Could you check a few things on this model? Use its own coordinates, in mm. Face numbers are marked on the shaded views. A direction names the side the tool comes from. Give positions to 0.01 mm unless a question says otherwise; leave off trailing zeros. Write each loop counter-clockwise with the first axis right and the second up, starting at its lowest first coordinate (ties: lowest second). Pieces come first, ordered by that corner, then holes. Notation, with made-up numbers: (48.5, 9.25) - (71.5, 9.25) arc R23 cw to (71.5, 42.25) - close; hole circle Ø7 at (70, 23). An arc over 180 degrees is marked (long way). Answer as CSV lines item,"result". Start each with the question number.
Q1. Imagine slicing it at B-B on x = 23. List the corners of the cut face in (y, z) for me.
Q2. Imagine slicing it at A-A on z = 7.9. List the corners of the cut face in (x, y) for me.
Q3. We'd pull the mould along X, two halves only. Please class the marked faces 4, 5, 6 and 7: pulls with the +X half, pulls with the -X half, needs draft (parallel to the pull), parting line crosses it, or undercut.
Q4. On a 3-axis mill with a long thin cutter (end or side, diameter ignored), from which of +Z, -Z, +X, -X, +Y, -Y can I reach the whole of each face in a straight line? I mean the marked faces 1, 2 and 3. Say none if no direction works.
Q5. Imagine slicing it at D-D on z = -4. List the corners of the cut face in (x, y) for me, and give its area (3 significant figures).
Q6. If I drill on line 1 along Z through (x, y) = (20, -7); line 2 along X through (y, z) = (-11, 9); line 3 along Y through (x, z) = (12.5, 0.5), over which ranges is the centre line in solid material (lowest first)?
Q7. Will these pins go through, and if not, where does the flat tip stop? pin 1 Ø2 at (x, z) = (20, -6) entering from -Y; pin 2 Ø12 at (x, y) = (22, 2) entering from -Z; pin 3 Ø11 at (y, z) = (-1, -22) entering from +X.
Q8. Imagine slicing it at C-C on y = -12.7. List the corners of the cut face in (x, z) for me.
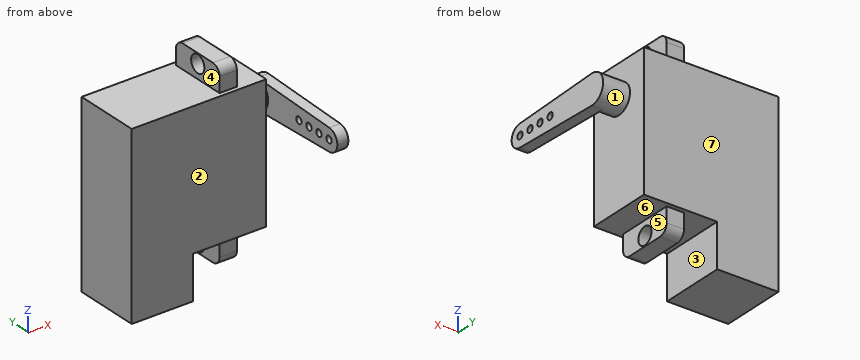
```python
from build123d import *

# Parameters (mm, degrees)
SKETCH1_W                          = 31
SKETCH1_H                          = 15.2
BOSS_EXTRUDE1_DEPTH                = 31
BOSS_EXTRUDE2_START                = 21
BOSS_EXTRUDE2_DEPTH                = 4
F_4_0MM_DOWEL_HOLE1_D              = 4
F_4_0MM_DOWEL_HOLE1_DEPTH          = 10.668
F_4_0MM_DOWEL_HOLE1_TIP            = 1.201721238
SKETCH6_R                          = 3.38413067
BOSS_EXTRUDE3_DEPTH                = 6.2
BOSS_EXTRUDE4_DEPTH                = 2.54
F_1_16_0_0625_DIAMETER_HOLE1_D     = 1.5875
F_1_16_0_0625_DIAMETER_HOLE1_DEPTH = 2.54
SKETCH12_W                         = 14.1
SKETCH12_H                         = 15.2
BOSS_EXTRUDE5_DEPTH                = 10


with BuildPart() as part:
    # Sketch1 → Boss-Extrude1 (new body)
    with BuildSketch(Plane(origin=(0, 0, 0), x_dir=(0, 0, -1), z_dir=(1, 0, 0))):
        Rectangle(SKETCH1_W, SKETCH1_H)
    extrude(amount=BOSS_EXTRUDE1_DEPTH)

    # Sketch2 → Boss-Extrude2 (add)
    with BuildSketch(Plane(origin=(0, 0, 0), x_dir=(0, 0, -1), z_dir=(1, 0, 0)).offset(BOSS_EXTRUDE2_START)):
        with BuildLine():
            Line((-15.5, 6.6), (-19, 6.6))
            ThreePointArc((-19, 6.6), (-20.414213562, 6.014213562), (-21, 4.6))
            Line((-21, 4.6), (-21, -4.6))
            ThreePointArc((-21, -4.6), (-20.414213562, -6.014213562), (-19, -6.6))
            Line((-19, -6.6), (-15.5, -6.6))
            Line((-15.5, -6.6), (-15.5, 6.6))
        make_face()
        with BuildLine():
            Line((15.5, -6.6), (19, -6.6))
            ThreePointArc((19, -6.6), (20.414213562, -6.014213562), (21, -4.6))
            Line((21, -4.6), (21, 4.6))
            ThreePointArc((21, 4.6), (20.414213562, 6.014213562), (19, 6.6))
            Line((19, 6.6), (15.5, 6.6))
            Line((15.5, 6.6), (15.5, -6.6))
        make_face()
    extrude(amount=BOSS_EXTRUDE2_DEPTH)

    # Ø4.0mm Dowel Hole1
    with Locations(Plane(origin=(25, 0, 0), x_dir=(0, 0, -1), z_dir=(1, 0, 0))):
        with Locations((-18.75, 0), (18.75, 0)):
            Hole(F_4_0MM_DOWEL_HOLE1_D / 2, depth=F_4_0MM_DOWEL_HOLE1_DEPTH)
            with Locations((0, 0, -(F_4_0MM_DOWEL_HOLE1_DEPTH + F_4_0MM_DOWEL_HOLE1_TIP / 2))):  # 118° drill point
                Cone(0, F_4_0MM_DOWEL_HOLE1_D / 2, F_4_0MM_DOWEL_HOLE1_TIP, mode=Mode.SUBTRACT)

    # Sketch6 → Boss-Extrude3 (add)
    with BuildSketch(Plane(origin=(31, 0, 0), x_dir=(0, 0, -1), z_dir=(1, 0, 0))):
        with Locations((-7.9, 0)):
            Circle(SKETCH6_R)
    extrude(amount=BOSS_EXTRUDE3_DEPTH)

    # Sketch7 → Boss-Extrude4 (add)
    with BuildSketch(Plane(origin=(37.2, 0, 0), x_dir=(0, 0, -1), z_dir=(1, 0, 0))):
        with BuildLine():
            Line((-4.518397081, -0.130774972), (-5.361897234, -21.942154729))
            ThreePointArc((-5.361897234, -21.942154729), (-7.9, -24.384), (-10.438102766, -21.942154729))
            Line((-10.438102766, -21.942154729), (-11.281602919, -0.130774972))
            ThreePointArc((-11.281602919, -0.130774972), (-7.9, 3.38413067), (-4.518397081, -0.130774972))
        make_face()
    extrude(amount=-BOSS_EXTRUDE4_DEPTH)

    # 1/16 (0.0625) Diameter Hole1
    with Locations(Plane(origin=(37.2, 0, 0), x_dir=(0, 0, -1), z_dir=(1, 0, 0))):
        with Locations((-7.9, -12.7), (-7.9, -15.748), (-7.9, -18.796), (-7.9, -21.844)):
            Hole(F_1_16_0_0625_DIAMETER_HOLE1_D / 2, depth=F_1_16_0_0625_DIAMETER_HOLE1_DEPTH)

    # Sketch12 → Boss-Extrude5 (add)
    with BuildSketch(Plane(origin=(0, 0, -15.5), x_dir=(-1, 0, 0), z_dir=(0, 0, -1))):
        with Locations((-7.05, 0)):
            Rectangle(SKETCH12_W, SKETCH12_H)
    extrude(amount=BOSS_EXTRUDE5_DEPTH)


solid = part.part
```
Conclusion:
1,outline,"(-7.6, -15.5) - (-6.6, -15.5) - (-6.6, -19) arc R2 ccw to (-4.6, -21) - (4.6, -21) arc R2 ccw to (6.6, -19) - (6.6, -15.5) - (7.6, -15.5) - (7.6, 15.5) - (6.6, 15.5) - (6.6, 19) arc R2 ccw to (4.6, 21) - (-4.6, 21) arc R2 ccw to (-6.6, 19) - (-6.6, 15.5) - (-7.6, 15.5) - close; hole circle Ø4 at (0, -18.75); hole circle Ø4 at (0, 18.75)"
2,outline,"(0, -7.6) - (31, -7.6) - (31, -3.38) - (34.66, -3.38) - (34.66, -11.91) - (37.2, -11.91) - (37.2, 3.38) - (31, 3.38) - (31, 7.6) - (0, 7.6) - close; (34.66, -24.38) - (37.2, -24.38) - (37.2, -22.64) - (34.66, -22.64) - close; (34.66, -21.05) - (37.2, -21.05) - (37.2, -19.59) - (34.66, -19.59) - close; (34.66, -18) - (37.2, -18) - (37.2, -16.54) - (34.66, -16.54) - close; (34.66, -14.95) - (37.2, -14.95) - (37.2, -13.49) - (34.66, -13.49) - close"
3,face 4,"pulls with the -X half"
3,face 5,"pulls with the +X half"
3,face 6,"undercut"
3,face 7,"needs draft"
4,face 1,"none"
4,face 2,"+Z, -Z, -X, -Y"
4,face 3,"-Z, +Y, -Y"
5,outline,"(0, -7.6) - (31, -7.6) - (31, 7.6) - (0, 7.6) - close"
5,area,"471 mm^2"
6,line 1,"-15.5 to 15.5"
6,line 2,"34.66 to 37.2"
6,line 3,"-7.6 to 7.6"
7,pin 1,"y = -7.6"
7,pin 2,"z = -21"
7,pin 3,"x = 25"
8,outline,"(34.66, 5) - (37.2, 5) - (37.2, 7.11) - (34.66, 7.11) - close; (34.66, 8.69) - (37.2, 8.69) - (37.2, 10.8) - (34.66, 10.8) - close"
